The model under review builds one solid part; all positions refer to its coordinate system, in mm. Round coordinates to 2 decimals unless told otherwise and drop trailing zeros. Loops run counter-clockwise (first coordinate to the right, second up) from the corner with the lowest first, then second, coordinate; pieces in that order, holes last. Notation, with made-up numbers: (62, 71) -> (76, 71) arc R16 ccw to (76, 78) -> close; hole circle Ø7 at (32.5, -29). An arc over 180 degrees is marked (long way). Use a Markdown table: item, result. Add a question column.
1) Insertion check: pin 1 (6.5 mm diameter, centred on x = 19.62, z = 3.24, fed in from -Y); pin 2 (1 mm diameter, centred on x = 28.5, z = -9.5, fed in from -Y). Each pin has a flat end and moves straight along its axis. Give the tip position at first contact, or say it passes through.
2) Consider section D-D on z = -3.5. Give the boundary of the cut face in (x, y), plus the area to 3 significant figures.
3) Consider section C-C on x = 9. Give the boundary of the cut face in (y, z).
4) Consider section B-B on y = 0.1. Give the boundary of the cut face in (x, z), plus the area to 3 significant figures.
5) Consider section A-A on x = 22.5. Give the boundary of the cut face in (y, z), plus the area to 3 significant figures.
6) Wall thickness on probe 1 along X at (y, z) = (0.4, 1); probe 2 along X at (y, z) = (0.3, -3); probe 3 along X at (y, z) = (0.4, -2): over which ranges is each line inside the solid? List them lowest first.
from build123d import *

# Parameters (mm, degrees)
SALIENTE_EXTRUIR2_DEPTH = 0.5
CORTAR_EXTRUIR1_DEPTH   = 0.5
SALIENTE_EXTRUIR3_DEPTH = 0.5


with BuildPart() as part:
    # Croquis2 → Saliente-Extruir2 (new body)
    with BuildSketch(Plane(origin=(0, 0, 0), x_dir=(1, 0, 0), z_dir=(0, 1, 0))):
        with BuildLine():
            Line((0, 0), (20, 0))
            Line((20, 0), (39.463577456, -4.600994744))
            ThreePointArc((39.463577456, -4.600994744), (39.040324802, 2.548287638), (34.753818463, 8.285642846))
            ThreePointArc((34.753818463, 8.285642846), (21.920955681, 16.476389899), (7.548005539, 11.457524625))
            ThreePointArc((7.548005539, 11.457524625), (2.056591074, 6.860161407), (0, 0))
        make_face()
    extrude(amount=SALIENTE_EXTRUIR2_DEPTH)

    # Croquis3 → Cortar-Extruir1 (cut)
    with BuildSketch(Plane(origin=(0, 0.5, 0), x_dir=(1, 0, 0), z_dir=(0, 1, 0))):
        with BuildLine():
            Line((20, 0), (16.5, 0))
            ThreePointArc((16.5, 0), (20.143291885, 1.229040833), (23.406126055, -0.80517408))
            Line((23.406126055, -0.80517408), (20, 0))
        make_face()
    extrude(amount=-CORTAR_EXTRUIR1_DEPTH, mode=Mode.SUBTRACT)

    # Croquis4 → Saliente-Extruir3 (add)
    with BuildSketch(Plane(origin=(0, 0.5, 0), x_dir=(1, 0, 0), z_dir=(0, 1, 0))):
        with BuildLine():
            Line((-0.246717473, -2.116141109), (16.897027571, -6.168750709))
            ThreePointArc((16.897027571, -6.168750709), (18.02539366, 0.426780522), (23.62217394, -3.240683553))
            ThreePointArc((23.62217394, -3.240683553), (23.080050106, -5.251427798), (21.600627731, -6.717135853))
            Line((21.600627731, -6.717135853), (39.216859982, -6.717135853))
            Line((39.216859982, -6.717135853), (39.463577456, -4.600994744))
            Line((39.463577456, -4.600994744), (20.690616261, 2.904236285))
            Line((20.690616261, 2.904236285), (0, 0))
            Line((0, 0), (-0.246717473, -2.116141109))
        make_face()
    extrude(amount=-SALIENTE_EXTRUIR3_DEPTH)


solid = part.part
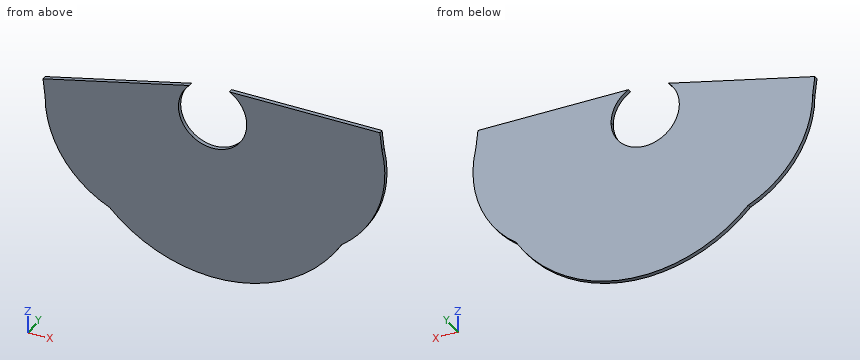
Result set:
| question | item | result |
|---|---|---|
| 1 | pin 1 | through |
| 1 | pin 2 | y = 0 |
| 2 | outline | (0.5, 0) -> (38.65, 0) -> (38.65, 0.5) -> (0.5, 0.5) -> close |
| 2 | area | 19.1 mm2 |
| 3 | outline | (0, -12.76) -> (0.5, -12.76) -> (0.5, 4.3) -> (0, 4.3) -> close |
| 4 | outline | (-0.25, 2.12) -> (0, 0) arc R12.47 ccw to (7.55, -11.46) arc R17.43 ccw to (34.75, -8.29) arc R12.47 ccw to (39.46, 4.6) -> (39.22, 6.72) -> (21.6, 6.72) arc R4 cw (long way) to (16.9, 6.17) -> close |
| 4 | area | 659 mm2 |
| 5 | outline | (0, -16.4) -> (0.5, -16.4) -> (0.5, 0.46) -> (0, 0.46) -> close; (0, 6.02) -> (0.5, 6.02) -> (0.5, 6.72) -> (0, 6.72) -> close |
| 5 | area | 8.78 mm2 |
| 6 | probe 1 | -0.12 to 16.31, 22.94 to 39.78 |
| 6 | probe 2 | 0.37 to 38.87 |
| 6 | probe 3 | 0.16 to 39.23 |
